Check sheet for the drawn part. Datum: minimum x, y, z corner. Units: mm. Round coordinates to 2 decimals unless told otherwise and drop trailing zeros. Write each loop counter-clockwise with the first axis right and the second up, starting at its lowest first coordinate (ties: lowest second). Pieces come first, ordered by that corner, then holes.
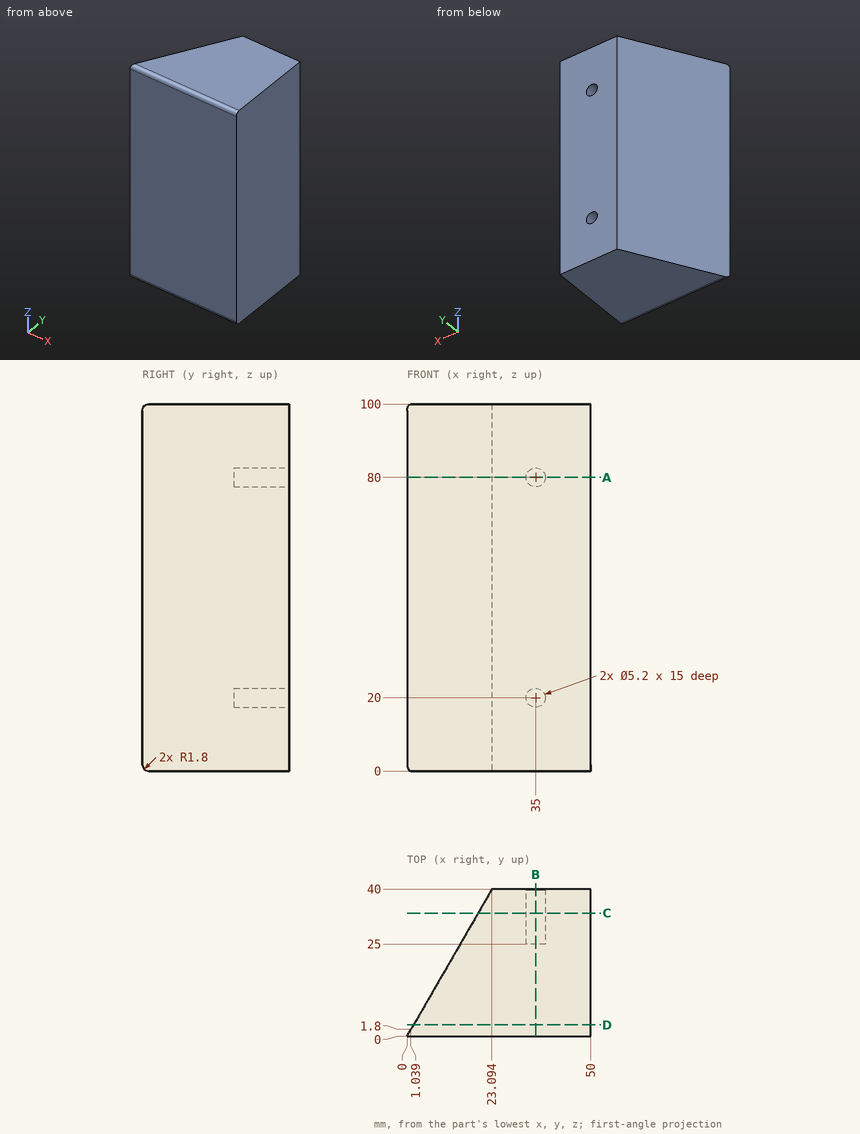
Q1. Sectioned sample at C-C (y = 33.5). Enter the section's corners in (x, z), plus the area to 3 significant figures.
Recorded:
outline: (19.34, 0) - (50, 0) - (50, 100) - (19.34, 100) - close; hole circle Ø5.2 at (35, 20); hole circle Ø5.2 at (35, 80)
area: 3,020 mm2
Q2. Sectioned sample at A-A (z = 80). Enter the section's corners in (x, y), plus the area to 3 significant figures.
Recorded:
outline: (0, 0) - (50, 0) - (50, 40) - (37.6, 40) - (37.6, 25) - (32.4, 25) - (32.4, 40) - (23.09, 40) - close
area: 1,460 mm2
Q3. Sectioned sample at B-B (x = 35). Enter the section's corners in (y, z), plus the area to 3 significant figures.
Recorded:
outline: (0, 1.8) arc R1.8 ccw to (1.8, 0) - (40, 0) - (40, 17.4) - (25, 17.4) - (25, 22.6) - (40, 22.6) - (40, 77.4) - (25, 77.4) - (25, 82.6) - (40, 82.6) - (40, 100) - (1.8, 100) arc R1.8 ccw to (0, 98.2) - close
area: 3,840 mm2
Q4. Sectioned sample at D-D (y = 3). Enter the section's corners in (x, z), plus the area to 3 significant figures.
Recorded:
outline: (1.73, 0) - (50, 0) - (50, 100) - (1.73, 100) - close
area: 4,830 mm2
Q5. Material ranges on line 1 along Z through (x, y) = (35, 36.25); line 2 along Z through (x, y) = (34, 36); line 3 along X through (y, z) = (31.25, 80), recorded low to high.
Recorded:
line 1: z = 0 to 17.4, 22.6 to 77.4, 82.6 to 100
line 2: z = 0 to 17.6, 22.4 to 77.6, 82.4 to 100
line 3: x = 18.04 to 32.4, 37.6 to 50
Q6. Depth check by flat-ended pin: P1, Ø3, axis at x = 38, z = 68.5, coming from the -Y side; P2, Ø10, axis at y = 36, z = 75.5, coming from the -X side; P3, Ø8, axis at x = 18.5, z = 87.5, coming from the +Y side; P4, Ø3, axis at y = 12.5, z = 11.5, coming from the -X side. Enter the tip coordinate at first touch or a pass-through.
Recorded:
P1: stops at y = 0
P2: stops at x = 17.9
P3: stops at y = 38.97
P4: stops at x = 6.35
